Input: part model. Units: mm. Frame: model coordinates. Give positions to 0.01 mm unless a question says otherwise; leave off trailing zeros. Loops run counter-clockwise (first coordinate to the right, second up) from the corner with the lowest first, then second, coordinate; pieces in that order, holes last. Notation, with made-up numbers: (50.25, 80) - (66.25, 80) arc R22 cw to (66.25, 111) - close; hole circle Ø6 at (14, 83.5). An arc over 180 degrees is marked (long way). Answer as a JSON object with one key per item and string values.
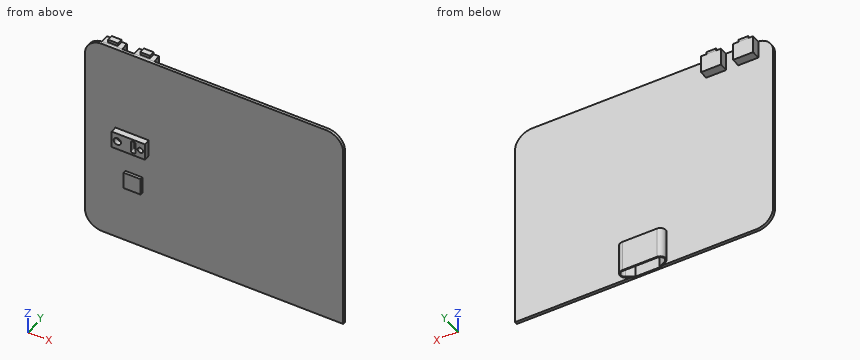
from build123d import *

# Parameters (mm, degrees)
SKETCH_1_W          = 45
SKETCH_1_H          = 36.5
EXTRUDE_1_DEPTH     = 0.5
FILLET_1_R          = 3
SKETCH_2_W          = 5.8
SKETCH_2_H          = 3
EXTRUDE_2_DEPTH     = 1.1
SKETCH_3_R          = 0.65
SKETCH_3_R_2        = 0.47
CUT_EXTRUDE_1_DEPTH = 0.9
FILLET_2_R          = 0.1
SKETCH_4_W          = 3
SKETCH_4_H          = 3
EXTRUDE_3_DEPTH     = 0.5
SKETCH_5_W          = 8
SKETCH_5_H          = 5.5
EXTRUDE_4_DEPTH     = 2.5
FILLET_3_R          = 1
CUT_EXTRUDE_2_DEPTH = 39.704941545
FILLET_4_R          = 1
CUT_EXTRUDE_3_DEPTH = 4.5
SKETCH_9_W          = 3.5
SKETCH_9_H          = 3.1
EXTRUDE_5_DEPTH     = 1.5
SKETCH_10_W         = 1.7
SKETCH_10_H         = 1
EXTRUDE_6_DEPTH     = 0.5


with BuildPart() as part:
    # Эскиз1 → Бобышка-Вытянуть1 (new body)
    with BuildSketch(Plane(origin=(0, 0, 0), x_dir=(1, 0, 0), z_dir=(0, 1, 0))):
        Rectangle(SKETCH_1_W, SKETCH_1_H)
    extrude(amount=EXTRUDE_1_DEPTH)

    # Скругление1
    fillet_1_edges = [part.edges().sort_by_distance(p)[0] for p in [
        (22.5, 0.25, 18.25),
        (-22.5, 0.25, 18.25),
        (-22.5, 0.25, -18.25),
    ]]
    fillet(fillet_1_edges, radius=FILLET_1_R)

    # Эскиз2 → Бобышка-Вытянуть2 (add)
    with BuildSketch(Plane.XZ):
        with Locations((-14.3, 1.45)):
            Rectangle(SKETCH_2_W, SKETCH_2_H)
    extrude(amount=EXTRUDE_2_DEPTH)

    # Эскиз3 → Вырез-Вытянуть1 (cut)
    with BuildSketch(Plane.XZ.offset(1.1)):
        with Locations(Location((-16.2, 1.45, 0), (0, 0, 270))):
            Circle(SKETCH_3_R)
        with Locations(Location((-12.2, 1.45, 0), (0, 0, 270))):
            Circle(SKETCH_3_R_2)
        with BuildLine():
            Line((-13.66, 2.55), (-13.26, 2.55))
            ThreePointArc((-13.26, 2.55), (-13.118578644, 2.491421356), (-13.06, 2.35))
            Line((-13.06, 2.35), (-13.06, 0.55))
            ThreePointArc((-13.06, 0.55), (-13.118578644, 0.408578644), (-13.26, 0.35))
            Line((-13.26, 0.35), (-13.66, 0.35))
            ThreePointArc((-13.66, 0.35), (-13.801421356, 0.408578644), (-13.86, 0.55))
            Line((-13.86, 0.55), (-13.86, 2.35))
            ThreePointArc((-13.86, 2.35), (-13.801421356, 2.491421356), (-13.66, 2.55))
        make_face()
    extrude(amount=-CUT_EXTRUDE_1_DEPTH, mode=Mode.SUBTRACT)

    # Скругление2
    fillet_2_edges = [part.edges().sort_by_distance(p)[0] for p in [
        (-13.801421356, -0.2, 0.408578644),
        (-13.86, -0.2, 1.45),
        (-13.801421356, -0.2, 2.491421356),
        (-13.46, -0.2, 2.55),
        (-13.118578644, -0.2, 2.491421356),
        (-13.06, -0.2, 1.45),
        (-13.118578644, -0.2, 0.408578644),
        (-13.46, -0.2, 0.35),
    ]]
    fillet(fillet_2_edges, radius=FILLET_2_R)

    # Эскиз4 → Бобышка-Вытянуть3 (add)
    with BuildSketch(Plane.XZ):
        with Locations((-14, -6.25)):
            Rectangle(SKETCH_4_W, SKETCH_4_H)
    extrude(amount=EXTRUDE_3_DEPTH)

    # Эскиз5 → Бобышка-Вытянуть4 (add)
    with BuildSketch(Plane(origin=(0, 0.5, 0), x_dir=(1, 0, 0), z_dir=(0, 1, 0))):
        with Locations((-0.7, 15.85)):
            Rectangle(SKETCH_5_W, SKETCH_5_H)
    extrude(amount=EXTRUDE_4_DEPTH)

    # Скругление3
    fillet_3_edges = [part.edges().sort_by_distance(p)[0] for p in [
        (3.3, 3, -15.85),
        (-4.7, 3, -15.85),
    ]]
    fillet(fillet_3_edges, radius=FILLET_3_R)

    # Эскиз6 → Вырез-Вытянуть2 (cut, through all)
    with BuildSketch(Plane.XY.offset(-13.1)):
        Polygon((-4.7, 0.5), (-2.816810686, 0.5), (-4.7, 1.540058106), align=None)
        Polygon((3.3, 1.540058106), (1.416810686, 0.5), (3.3, 0.5), align=None)
    extrude(amount=-CUT_EXTRUDE_2_DEPTH, mode=Mode.SUBTRACT)

    # Скругление4
    # the kernel refuses this fillet: 1 mm, written as the material it takes off along each edge
    with BuildSketch(Plane(origin=(3.3, 1.540058106, -11.651007536), x_dir=(-0.8753697639222053, -0.48345400651021836, 0), z_dir=(0, 0, -1))) as fillet_4_piece_1:
        with BuildLine():
            CenterArc((0.579596986, 1), FILLET_4_R, 216.682538738, 53.317461262)
            Line((-0.222360751, 0.402619227), (-0.238399906, 0.390671612))
            ThreePointArc((-0.238399906, 0.390671612), (-0.128687771, 0.191640533), (-0.017507395, -0.00966908))
            Line((-0.017507395, -0.00966908), (0, -0.02))
            Line((0, -0.02), (0.579596986, -0.02))
            Line((0.579596986, -0.02), (0.579596986, 0))
        make_face()
    extrude(amount=8.397984929, mode=Mode.SUBTRACT)
    with BuildSketch(Plane(origin=(-4.7, 1.540058106, -11.651007536), x_dir=(0, 1, 0), z_dir=(0, 0, -1))) as fillet_4_piece_2:
        with BuildLine():
            CenterArc((0.595161279, 0.990815683), FILLET_4_R, 208.911232689, 53.317461262)
            Line((-0.280208485, 0.507361677), (-0.29771588, 0.497692596))
            Line((-0.29771588, 0.497692596), (-0.017507395, -0.00966908))
            Line((-0.017507395, -0.00966908), (0, -0.02))
            ThreePointArc((0, -0.02), (0.229970947, -0.02), (0.457237506, -0.019816314))
            Line((0.457237506, -0.019816314), (0.459941894, 0))
        make_face()
    extrude(amount=8.397984929, mode=Mode.SUBTRACT)

    # Эскиз8 → Вырез-Вытянуть3 (cut)
    with BuildSketch(Plane(origin=(0, 0, -18.6), x_dir=(-1, 0, 0), z_dir=(0, 0, -1))):
        with BuildLine():
            Line((-2.695947522, 1.434923574), (-1.365252427, 0.7))
            Line((-1.365252427, 0.7), (2.765252427, 0.7))
            Line((2.765252427, 0.7), (4.095947522, 1.434923574))
            ThreePointArc((4.095947522, 1.434923574), (4.365171631, 1.677310395), (4.499884525, 2.013592163))
            ThreePointArc((4.499884525, 2.013592163), (4.260859282, 2.57047074), (3.7, 2.8))
            Line((3.7, 2.8), (-2.3, 2.8))
            ThreePointArc((-2.3, 2.8), (-2.860859282, 2.57047074), (-3.099884525, 2.013592163))
            ThreePointArc((-3.099884525, 2.013592163), (-2.965171631, 1.677310395), (-2.695947522, 1.434923574))
        make_face()
    extrude(amount=-CUT_EXTRUDE_3_DEPTH, mode=Mode.SUBTRACT)

    # Эскиз9 → Бобышка-Вытянуть5 (add)
    with BuildSketch(Plane(origin=(0, 0.5, 0), x_dir=(1, 0, 0), z_dir=(0, 1, 0))):
        with Locations((-18.15, -16.6)):
            Rectangle(SKETCH_9_W, SKETCH_9_H)
        with Locations((-12.55, -16.6)):
            Rectangle(SKETCH_9_W, SKETCH_9_H)
    extrude(amount=EXTRUDE_5_DEPTH)

    # Эскиз10 → Бобышка-Вытянуть6 (add)
    with BuildSketch(Plane.XY.offset(18.15)):
        with Locations((-18.15, 1.4)):
            Rectangle(SKETCH_10_W, SKETCH_10_H)
        with Locations((-12.55, 1.4)):
            Rectangle(SKETCH_10_W, SKETCH_10_H)
    extrude(amount=EXTRUDE_6_DEPTH)


solid = part.part
Item 1: Material intervals for line 1 (X direction, y = -0.55, z = 1.45); line 2 (Z direction, x = -14.5, y = -0.1); line 3 (X direction, y = 1.5, z = 16), sorted ascending. Write a range as [from, to].
Geometry check:
{"line 1": "x = [-17.2, -16.85], [-15.55, -13.86], [-13.06, -12.67], [-11.73, -11.4]", "line 2": "z = [-7.75, -4.75], [-0.05, 2.95]", "line 3": "x = [-19.9, -16.4], [-14.3, -10.8]"}
Item 2: Cut plane D-D (x = 19). Return loops of the section in (y, z).
Geometry check:
{"outline": "(0, -18.25) - (0.5, -18.25) - (0.5, 18.25) - (0, 18.25) - close"}
Item 3: Cut plane C-C (z = 16.5). Return loops of the section in (x, y), then the cut area to 3 significant figures.
Geometry check:
{"outline": "(-22.23, 0) - (22.23, 0) - (22.23, 0.5) - (-10.8, 0.5) - (-10.8, 2) - (-14.3, 2) - (-14.3, 0.5) - (-16.4, 0.5) - (-16.4, 2) - (-19.9, 2) - (-19.9, 0.5) - (-22.23, 0.5) - close", "area": "32.7 mm2"}
Item 4: Contact query for flat-ended pins moving along their axis: P1, Ø1, axis at x = -8.5, y = 0, coming from the -Z side; P2, Ø8, axis at x = -18, z = -7, coming from the +Y side; P3, Ø1.5, axis at y = 2, z = -0.5, coming from the -X side; P4, Ø2.5, axis at x = -19, z = 16.5, coming from the +Y side. Output: stop coordinate, or through.
Geometry check:
{"P1": "stops at z = -18.25", "P2": "stops at y = 0.5", "P3": "passes through", "P4": "stops at y = 2"}
Item 5: Cut plane B-B (z = 1.45). Return loops of the section in (x, y).
Geometry check:
{"outline": "(-22.5, 0) - (-17.2, 0) - (-17.2, -1.1) - (-16.85, -1.1) - (-16.85, -0.2) - (-15.55, -0.2) - (-15.55, -1.1) - (-13.86, -1.1) - (-13.86, -0.3) arc R0.1 cw to (-13.76, -0.2) - (-13.16, -0.2) arc R0.1 cw to (-13.06, -0.3) - (-13.06, -1.1) - (-12.67, -1.1) - (-12.67, -0.2) - (-11.73, -0.2) - (-11.73, -1.1) - (-11.4, -1.1) - (-11.4, 0) - (22.5, 0) - (22.5, 0.5) - (-22.5, 0.5) - close"}
Item 6: Cut plane A-A (x = -1.5). Return loops of the section in (y, z), then the cut area to 4 significant figures.
Geometry check:
{"outline": "(0, -18.25) - (0.5, -18.25) - (0.5, -18.6) - (0.7, -18.6) - (0.7, -14.1) - (2.8, -14.1) - (2.8, -18.6) - (3, -18.6) - (3, -13.1) - (0.5, -13.1) - (0.5, 18.25) - (0, 18.25) - close", "area": "22.55 mm2"}
